Autodesk Inventor part; units mm, degrees
ref_plane "YZ Plane" through (0, 0, 0) normal (1, 0, 0) x (0, 1, 0)
ref_plane "XZ Plane" through (0, 0, 0) normal (0, 1, 0) x (-1, 0, 0)
ref_plane "XY Plane" through (0, 0, 0) normal (0, 0, 1) x (1, 0, 0)
sketch "スケッチ1" plane through (0, 0, 0) normal (0, 0, 1) x (1, 0, 0)
  circle A0 centre (54.6996, 44) radius 4
  line L0 (62.6996, 0) -> (65.6996, 0)
  circle A1 centre (-0.366, 91.8281) radius 4
  circle A2 centre (-0.366, 91.8281) radius 4
  circle A3 centre (54.6996, 44) radius 4
  line L1 (58.602, 44.878) -> (68.6996, 0)
  line L2 (2.257, 94.8481) -> (57.3226, 47.0199)
  line L3 (2.7488, 95.4143) -> (57.8144, 47.5861)
  line L4 (59.3337, 45.0427) -> (69.4313, 0.1646)
  circle A4 centre (54.6996, 44) radius 4.75
  line L5 (2.257, 94.8481) -> (2.7488, 95.4143)
  line L6 (68.6996, 0) -> (69.4313, 0.1646)
  point P0 (0, 0)
  dimension "d0" = 0.75
  dimension "d1" = 0.75
  dimension "d2" = 0.75
extrude "押し出し1" add sketch "スケッチ1" along normal blind 20 contours A0 L2 A4 L1 | A4 L4 L6 L1 | L2 L5 L3 A4 picked at (56.3248, 48.0683)
sketch "スケッチ2" plane through (2.7488, 95.4143, 20) normal (0.6557, 0.755, 0) x (0.755, -0.6557, 0)
  line L0 (72.9366, 20) -> (0, 20)
  line L1 (0, 20) -> (0, 0)
  line L2 (72.9366, 0) -> (0, 0)
  line L3 (72.9366, 20) -> (72.9366, 0)
  line L4 (5, 0) -> (5, 20)
  circle A0 centre (5, 6.25) radius 1.5
  line L5 (72.9366, 12.5) -> (0, 12.5)
  point P0 (60.4926, 20)
  dimension "d5" = 5
  dimension "d6" = 3
  dimension "d7" = 6.25
  dimension "d15" = 7.5
sketch "スケッチ3" plane through (59.3337, 45.0427, 20) normal (0.9756, 0.2195, 0) x (0, 0, -1)
  line L0 (20, -46) -> (20, 0)
  line L1 (20, 0) -> (0, 0)
  line L2 (0, -46) -> (0, 0)
  line L3 (20, -46) -> (0, -46)
  line L4 (0, -41) -> (20, -41)
  circle A0 centre (10, -41) radius 1.5
  point P0 (20, -30.9196)
  dimension "d8" = 5
  dimension "d9" = 3
  dimension "d10" = 10
extrude "押し出し2" cut sketch "スケッチ2" against normal blind 10 contours L3 L5 L4 L0 | L4 L5 L1 L0 | A0 L4 | L4 A0
extrude "押し出し3" cut sketch "スケッチ3" against normal blind 10 contours A0 L4 | L4 A0
properties part number "アームガードfull" material "ポリプロピレン"
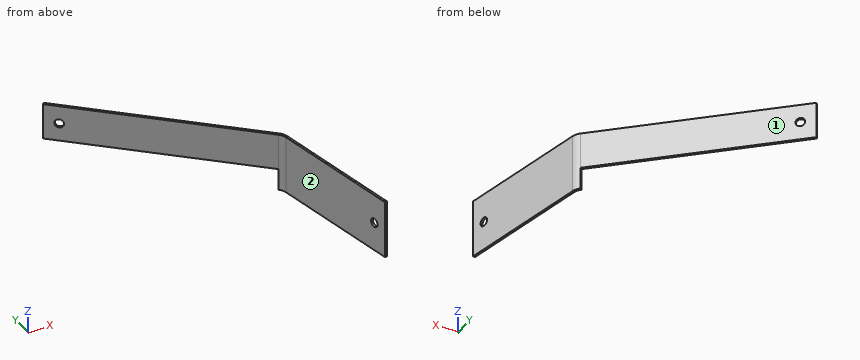
The listing builds one solid part. Answer for the finished solid, in the listing's coordinates (mm). Face numbers are marked on the shaded views. Coordinates: 2 decimals unless noted, no trailing zeros. Loops run counter-clockwise (first coordinate to the right, second up) from the corner with the lowest first, then second, coordinate; pieces in that order, holes last. Notation, with made-up numbers: (24, 14.25) -> (50, 14.25) arc R30 cw to (50, 40.25) -> close; hole circle Ø2 at (77, -18.5). An arc over 180 degrees is marked (long way). Write item = value, one per line. Start each with the question number.
1) The mould has two halves that part along Y. Classify the marked faces 1 and 2: released by +Y, released by -Y, zero draft, split by the parting line, or undercut.
2) Straight lines are drawn through the part: line 1 (X direction, y = 28, z = 7.25); line 2 (X direction, y = 20, z = 9.75); line 3 (Y direction, x = 21.5, z = 15.25). For each, find the intervals that lie inside material, in ascending order. Write a range as from..to.
3) A cutting plane is placed at C-C (x = 24). Give the vertices of the cut face in (y, z), then the cut area to 3 significant figures.
4) A cutting plane is placed at D-D (z = 3.5). Give the vertices of the cut face in (x, y), then the cut area to 3 significant figures.
5) A cutting plane is placed at A-A (z = 18.5). Give the vertices of the cut face in (x, y), then the cut area to 3 significant figures.
6) A cutting plane is placed at B-B (y = 25.5). Give the vertices of the cut face in (x, z), then the cut area to 3 significant figures.
7) Given pin 1 Ø3 at (x, z) = (42.5, 16.5) entering from -Y; pin 2 Ø8 at (x, z) = (46, 14) entering from -Y; pin 3 Ø4 at (x, z) = (26, 14.5) entering from -Y, each flat-ended and moving along its own axis, determine where each tip first touches the part or whether it passes through.
Responses:
q1.face_1 = released by +Y
q1.face_2 = released by -Y
q2.line_1 = 62.4..63.17
q2.line_2 = 64.2..64.97
q2.line_3 = 78.13..79.13
q3.outline = (75.96, 7.5) -> (76.96, 7.5) -> (76.96, 20) -> (75.96, 20) -> close
q3.area = 12.4 mm²
q4.outline = (57.32, 47.02) arc R4 cw to (58.6, 44.88) -> (68.7, 0) -> (69.43, 0.16) -> (59.33, 45.04) arc R4.75 ccw to (57.81, 47.59) -> close
q4.area = 36.6 mm²
q5.outline = (2.26, 94.85) -> (57.32, 47.02) arc R4 cw to (58.6, 44.88) -> (68.7, 0) -> (69.43, 0.16) -> (59.33, 45.04) arc R4.75 ccw to (57.81, 47.59) -> (2.75, 95.41) -> close
q5.area = 91.3 mm²
q6.outline = (62.96, 0) -> (63.73, 0) -> (63.73, 20) -> (62.96, 20) -> close
q6.area = 15.4 mm²
q7.pin_1 = 58.59
q7.pin_2 = 53.38
q7.pin_3 = 72.49
